Source: CAD feature listing. Evaluate the final solid. Frame: model axes, mm. Give positions to 0.01 mm unless a question says otherwise; leave off trailing zeros. Write each loop counter-clockwise with the first axis right and the second up, starting at its lowest first coordinate (ties: lowest second). Pieces come first, ordered by that corner, then holes. Notation, with made-up numbers: (62, 65) -> (85, 65) arc R22 cw to (85, 78) -> close; hole circle Ø6 at (59.5, -10.5). An arc over 180 degrees is marked (long way). Write item = value, one per line.
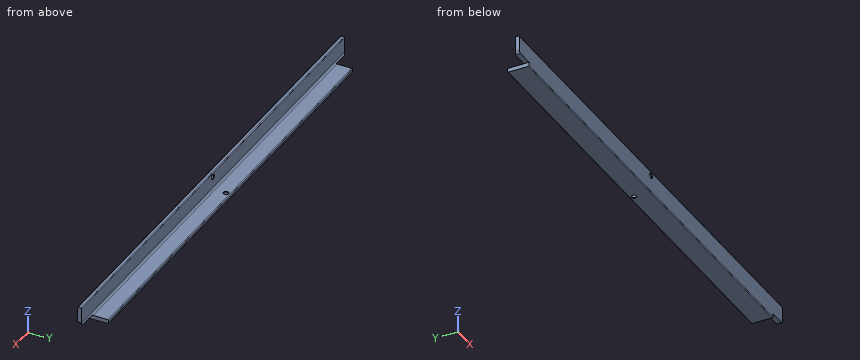
from build123d import *

# Parameters (mm, degrees)
F1_DEPTH  = 295
F2_R      = 1
F3_R      = 2.38125
F5_W      = 50
F5_H      = 50
F6_DEPTH  = 25
F7_R      = 2.5
F8_R      = 2.5
F9_DEPTH  = 25
F10_SIZE  = 0.5
F11_R     = 2.5
F12_DEPTH = 25
F13_SIZE  = 0.5


with BuildPart() as f1:
    # F0 (on Right) → F1 (new body, symmetric)
    with BuildSketch(Plane.YZ):
        Polygon((0, 25.4), (0, 0), (25.4, 0), (25.4, 4.7625), (4.7625, 4.7625), (4.7625, 25.4), align=None)
    extrude(amount=F1_DEPTH, both=True)

    # F2
    f2_edges = [f1.edges().sort_by_distance(p)[0] for p in [
        (0, 0, 25.4),
        (0, 4.7625, 25.4),
        (0, 0, 0),
        (0, 25.4, 4.7625),
        (0, 25.4, 0),
    ]]
    fillet(f2_edges, radius=F2_R)

    # F3
    f3_edges = [f1.edges().sort_by_distance(p)[0] for p in [
        (0, 4.7625, 4.7625),
    ]]
    fillet(f3_edges, radius=F3_R)

    # F5 (on face) → F6 (cut, symmetric)
    with BuildSketch(Plane(origin=(0, 4.7625, 0), x_dir=(-1, 0, 0), z_dir=(0, 1, 0))):
        with Locations((-298.5, -20)):
            Rectangle(F5_W, F5_H)
        with Locations((298.5, -20)):
            Rectangle(F5_W, F5_H)
    extrude(amount=F6_DEPTH, both=True, mode=Mode.SUBTRACT)

    # F7
    f7_edges = [f1.edges().sort_by_distance(p)[0] for p in [
        (295, 3.053539, 5),
        (-295, 3.053539, 5),
    ]]
    fillet(f7_edges, radius=F7_R)

    # F8 (on face) → F9 (cut)
    with BuildSketch(Plane.XY.offset(4.7625)):
        with Locations((0, 20)):
            Circle(F8_R)
    extrude(amount=-F9_DEPTH, mode=Mode.SUBTRACT)

    # F10
    f10_edges = [f1.edges().sort_by_distance(p)[0] for p in [
        (-2.5, 20, 4.7625),
        (2.5, 20, 2.38125),
        (-2.5, 20, 0),
    ]]
    chamfer(f10_edges, length=F10_SIZE)

    # F11 (on face) → F12 (cut)
    with BuildSketch(Plane.XZ):
        with Locations((0, 20)):
            Circle(F11_R)
    extrude(amount=-F12_DEPTH, mode=Mode.SUBTRACT)

    # F13
    f13_edges = [f1.edges().sort_by_distance(p)[0] for p in [
        (-2.5, 0, 20),
        (2.5, 2.38125, 20),
        (-2.5, 4.7625, 20),
    ]]
    chamfer(f13_edges, length=F13_SIZE)


solid = f1.part
1) Cut plane A-A (x = -214). Return the cut outline in (y, z), then the cut area to 3 significant figures.
Computed:
outline = (0, 1) arc R1 ccw to (1, 0) -> (24.4, 0) arc R1 ccw to (25.4, 1) -> (25.4, 3.76) arc R1 ccw to (24.4, 4.76) -> (7.14, 4.76) arc R2.38 cw to (4.76, 7.14) -> (4.76, 24.4) arc R1 ccw to (3.76, 25.4) -> (1, 25.4) arc R1 ccw to (0, 24.4) -> close
area = 219 mm²
2) Contact query for flat-ended pins moving along their axis: pin 1 (6 mm diameter, centred on x = -13.5, y = 16.5, fed in from +Z); pin 2 (8.5 mm diameter, centred on x = -110.5, z = 13.5, fed in from +Y); pin 3 (1.8 mm diameter, centred on x = -283, y = 3, fed in from -Z). Output: stop coordinate, or through.
Computed:
pin_1 = 4.76
pin_2 = 4.76
pin_3 = 5
3) Material intervals for L1, parallel to Y at x = 0, z = 3.5; L2, parallel to Y at x = 97.5, z = 9.75, sorted ascending.
Computed:
L1 = 0 to 17.5, 22.5 to 25.4
L2 = 0 to 4.76
